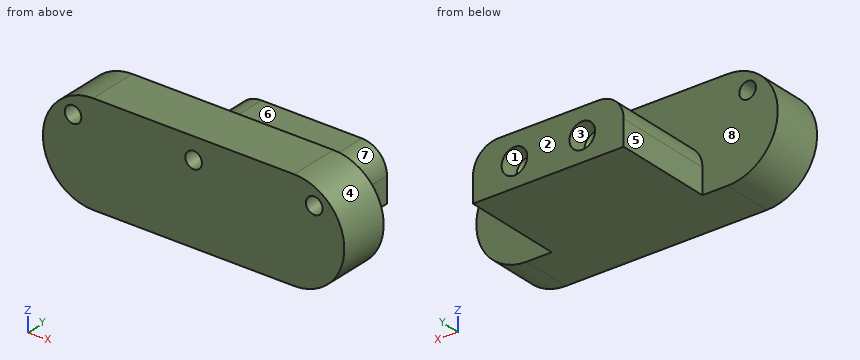
from build123d import *

# Parameters (mm, degrees)
BOSS_EXTRUDE1_DEPTH         = 10
TAP_DRILL_FOR_M4X0_7_TAP1_D = 3.3
SKETCH8_W                   = 30
SKETCH8_H                   = 10
BOSS_EXTRUDE2_DEPTH         = 20
FILLET1_R                   = 5
F_1_0MM_DOWEL_HOLE1_D       = 5.1
F_1_0MM_DOWEL_HOLE1_DEPTH   = 3.8
F_1_0MM_DOWEL_HOLE1_TIP     = 2.55


with BuildPart() as part:
    # Sketch3 → Boss-Extrude1 (new body)
    with BuildSketch(Plane(origin=(0, 0, 0), x_dir=(1, 0, 0), z_dir=(0, 1, 0))):
        with BuildLine():
            Line((-20, 10), (20, 10))
            ThreePointArc((20, 10), (30, 0), (20, -10))
            Line((20, -10), (-20, -10))
            ThreePointArc((-20, -10), (-30, 0), (-20, 10))
        make_face()
    extrude(amount=BOSS_EXTRUDE1_DEPTH)

    # Tap Drill for M4x0.7 Tap1 (through all)
    with Locations(Plane(origin=(0, 10, 0), x_dir=(1, 0, 0), z_dir=(0, 1, 0))):
        with Locations((0, -5.741156808), (24, -5.741156808), (-24, -5.741156808)):
            Hole(TAP_DRILL_FOR_M4X0_7_TAP1_D / 2)

    # Sketch8 → Boss-Extrude2 (add)
    with BuildSketch(Plane(origin=(0, 10, 0), x_dir=(1, 0, 0), z_dir=(0, 1, 0))):
        with Locations((0, 5)):
            Rectangle(SKETCH8_W, SKETCH8_H)
    extrude(amount=BOSS_EXTRUDE2_DEPTH)

    # Fillet1
    fillet1_edges = [part.edges().sort_by_distance(p)[0] for p in [
        (-15, 20, 0),
        (15, 20, 0),
    ]]
    fillet(fillet1_edges, radius=FILLET1_R)

    # Ø1.0mm Dowel Hole1
    with Locations(Plane(origin=(0, 30, 0), x_dir=(1, 0, 0), z_dir=(0, 1, 0))):
        with Locations((-6.75, 5.194379969), (6.75, 5.194379969)):
            Hole(F_1_0MM_DOWEL_HOLE1_D / 2, depth=F_1_0MM_DOWEL_HOLE1_DEPTH)
            with Locations((0, 0, -(F_1_0MM_DOWEL_HOLE1_DEPTH + F_1_0MM_DOWEL_HOLE1_TIP / 2))):  # 90° drill point
                Cone(0, F_1_0MM_DOWEL_HOLE1_D / 2, F_1_0MM_DOWEL_HOLE1_TIP, mode=Mode.SUBTRACT)


solid = part.part
CAD build for the part. Positions are in the model's coordinates, mm. Face numbers are marked on the shaded views. A direction names the side the tool comes from. Round coordinates to 2 decimals unless told otherwise and drop trailing zeros. Write each loop counter-clockwise with the first axis right and the second up, starting at its lowest first coordinate (ties: lowest second). Pieces come first, ordered by that corner, then holes.
(1) Slice it at A-A, the plane x = 0. Write the cut outline in (y, z), and give its area (3 significant figures).
(2) Slice it at C-C, the plane x = -16.5. Write the cut outline in (y, z).
(3) Probe line 1 along Z through (x, y) = (-6.75, 29); line 2 along X through (y, z) = (6.5, 5.5); line 3 along X through (y, z) = (8, 7). List the from-to ranges inside material, lowest first.
(4) 3-axis set-ups, long thin cutter, end or side, ignore diameter. For the marked faces 5, 6, 7 and 8: which of +Z, -Z, +X, -X, +Y, -Y reach the whole face in a straight line?
(5) Mould opens along Z. For the marked faces 1, 2, 3 and 4 say: pulls with the +Z half, pulls with the -Z half, needs draft (parallel to the pull), parting line crosses it, or undercut.
(6) Drop flat-ended pins along their axis: P1, Ø1.5, axis at x = -5, y = 22, coming from the +Z side; P2, Ø4, axis at y = 13.5, z = -2.5, coming from the -X side; P3, Ø6, axis at x = -13.5, z = 6.5, coming from the +Y side. Give the stop position or say it passes through.
(7) Slice it at B-B, the plane y = 22.25. Write the cut outline in (x, z), and give its area (3 significant figures).
(8) Slice it at D-D, the plane y = 8.5. Write the cut outline in (x, z).
From the geometry:
1. outline: (0, -10) - (30, -10) - (30, 0) - (10, 0) - (10, 4.09) - (0, 4.09) - close; (0, 7.39) - (10, 7.39) - (10, 10) - (0, 10) - close
1. area: 367 mm2
2. outline: (0, -10) - (10, -10) - (10, 10) - (0, 10) - close
3. line 1: z = -10 to -7.74, -2.64 to 0
3. line 2: x = -28.35 to -25.63, -22.37 to -1.63, 1.63 to 22.37, 25.63 to 28.35
3. line 3: x = -27.14 to -25.07, -22.93 to -1.07, 1.07 to 22.93, 25.07 to 27.14
4. face 5: +Z, -Z, -X, +Y
4. face 6: +Z, +X, -X, +Y
4. face 7: +Z, +X, +Y
4. face 8: +Z, +Y
5. face 1: undercut
5. face 2: needs draft
5. face 3: undercut
5. face 4: parting line crosses it
6. P1: stops at z = 0
6. P2: stops at x = -14.97
6. P3: stops at y = 10
7. outline: (-15, -10) - (15, -10) - (15, -5) arc R5 ccw to (10, 0) - (-10, 0) arc R5 ccw to (-15, -5) - close
7. area: 289 mm2
8. outline: (-20, -10) - (20, -10) arc R10 ccw to (20, 10) - (-20, 10) arc R10 ccw to start; hole circle Ø3.3 at (-24, 5.74); hole circle Ø3.3 at (0, 5.74); hole circle Ø3.3 at (24, 5.74)
